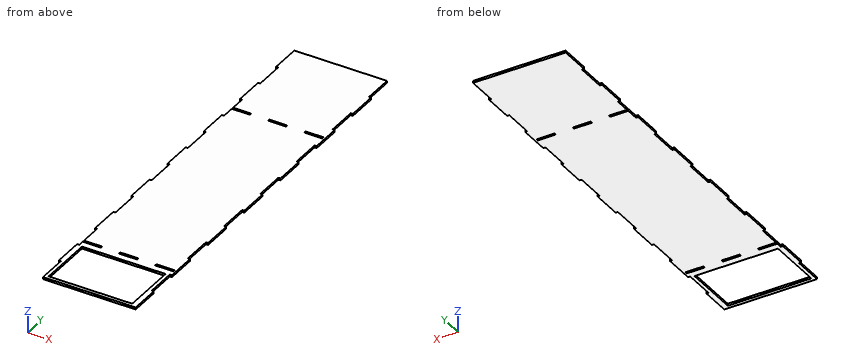
```python
from build123d import *

# Parameters (mm, degrees)
SKETCH1_W           = 120
SKETCH1_H           = 79
SKETCH1_W_2         = 26.12
SKETCH1_H_2         = 3
BOSS_EXTRUDE1_DEPTH = 3


with BuildPart() as part:
    # Sketch1 → Boss-Extrude1 (new body)
    with BuildSketch(Plane.XY):
        Polygon((65, 0), (-67.997818333, 0), (-67.997818333, -43.007142857), (-65, -43.007142857), (-65, -85.714285714), (-67.997818333, -85.714285714), (-67.997818333, -128.721428571), (-65, -128.721428571), (-65, -150), (-38.88, -150), (-38.88, -153), (-65, -153), (-65, -171.428571429), (-67.997818333, -171.428571429), (-67.997818333, -214.435714286), (-65, -214.435714286), (-65, -257.142857143), (-67.997818333, -257.142857143), (-67.997818333, -300.15), (-65, -300.15), (-65, -342.857142857), (-67.997818333, -342.857142857), (-67.997818333, -385.864285714), (-65, -385.864285714), (-65, -428.571428571), (-67.997818333, -428.571428571), (-67.997818333, -471.578571429), (-65, -471.578571429), (-65, -503), (-38.88, -503), (-38.88, -506), (-65, -506), (-65, -514.285714286), (-67.997818333, -514.285714286), (-67.997818333, -557.292857143), (-65, -557.292857143), (-65, -600), (67.997818333, -600), (67.997818333, -557.292857143), (65, -557.292857143), (65, -514.285714286), (67.997818333, -514.285714286), (67.997818333, -471.578571429), (65, -471.578571429), (65, -428.571428571), (67.997818333, -428.571428571), (67.997818333, -385.864285714), (65, -385.864285714), (65, -342.857142857), (67.997818333, -342.857142857), (67.997818333, -300.15), (65, -300.15), (65, -257.142857143), (67.997818333, -257.142857143), (67.997818333, -214.435714286), (65, -214.435714286), (65, -171.428571429), (67.997818333, -171.428571429), (67.997818333, -128.721428571), (65, -128.721428571), (65, -85.714285714), (67.997818333, -85.714285714), (67.997818333, -43.007142857), (65, -43.007142857), align=None)
        with Locations((0, -555.5)):
            Rectangle(SKETCH1_W, SKETCH1_H, mode=Mode.SUBTRACT)
        with Locations((0, -504.5)):
            Rectangle(SKETCH1_W_2, SKETCH1_H_2, mode=Mode.SUBTRACT)
        with Locations((51.94, -504.5)):
            Rectangle(SKETCH1_W_2, SKETCH1_H_2, mode=Mode.SUBTRACT)
        with Locations((0, -151.5)):
            Rectangle(SKETCH1_W_2, SKETCH1_H_2, mode=Mode.SUBTRACT)
        with Locations((51.94, -151.5)):
            Rectangle(SKETCH1_W_2, SKETCH1_H_2, mode=Mode.SUBTRACT)
    extrude(amount=BOSS_EXTRUDE1_DEPTH)


solid = part.part
```
Could you check a few things on this model? Use its own coordinates, in mm. Give positions to 0.01 mm unless a question says otherwise; leave off trailing zeros. Loops run counter-clockwise (first coordinate to the right, second up) from the corner with the lowest first, then second, coordinate; pieces in that order, holes last. Notation, with made-up numbers: (-25, -27) - (-19, -27) arc R17 ccw to (-19, -6) - close; hole circle Ø1 at (42.5, 69). An arc over 180 degrees is marked (long way). Answer in a Markdown table with one row per item. Add a question column.
Q1. If we section it at D-D (y = -452): List the corners of the cut face in (x, z) for me, plus the area to 3 significant figures.
Q2. Please list where these lines run through material, in increasing order: L1, parallel to Y at x = -41, z = 2.45; L2, parallel to X at y = -565, z = 1.35; L3, parallel to Y at x = -22, z = 1.75. Write a range as from..to.
Q3. If we section it at A-A (x = 46): List the corners of the cut face in (y, z) for me.
Q4. For pin 1 (0.9 mm diameter, centred on x = -67, z = 2, fed in from -Y); pin 2 (0.9 mm diameter, centred on x = -66, z = 2, fed in from +Y); pin 3 (1.5 mm diameter, centred on x = 66, z = 1.5, fed in from +Y), each with a flat end and sliding along its axis, tell me the tip position at first contact or that it passes through.
Q5. If we section it at B-B (x = -26.5): List the corners of the cut face in (y, z) for me, plus the area to 3 significant figures.
Q6. If we section it at C-C (z = 0.9): State how many separate pieces and enclosed holes the cut face has, plus the area to 3 significant figures.
The answers:
| question | item | result |
|---|---|---|
| 1 | outline | (-68, 0) - (65, 0) - (65, 3) - (-68, 3) - close |
| 1 | area | 399 mm^2 |
| 2 | L1 | y = -600..-595, -516..-506, -503..-153, -150..0 |
| 2 | L2 | x = -65..-60, 60..68 |
| 2 | L3 | y = -600..-595, -516..0 |
| 3 | outline | (-600, 0) - (-595, 0) - (-595, 3) - (-600, 3) - close; (-516, 0) - (-506, 0) - (-506, 3) - (-516, 3) - close; (-503, 0) - (-153, 0) - (-153, 3) - (-503, 3) - close; (-150, 0) - (0, 0) - (0, 3) - (-150, 3) - close |
| 4 | pin 1 | stops at y = -557.29 |
| 4 | pin 2 | stops at y = 0 |
| 4 | pin 3 | stops at y = -43.01 |
| 5 | outline | (-600, 0) - (-595, 0) - (-595, 3) - (-600, 3) - close; (-516, 0) - (0, 0) - (0, 3) - (-516, 3) - close |
| 5 | area | 1,560 mm^2 |
| 6 | separate pieces | 1 |
| 6 | enclosed holes | 5 |
| 6 | area | 69,800 mm^2 |
